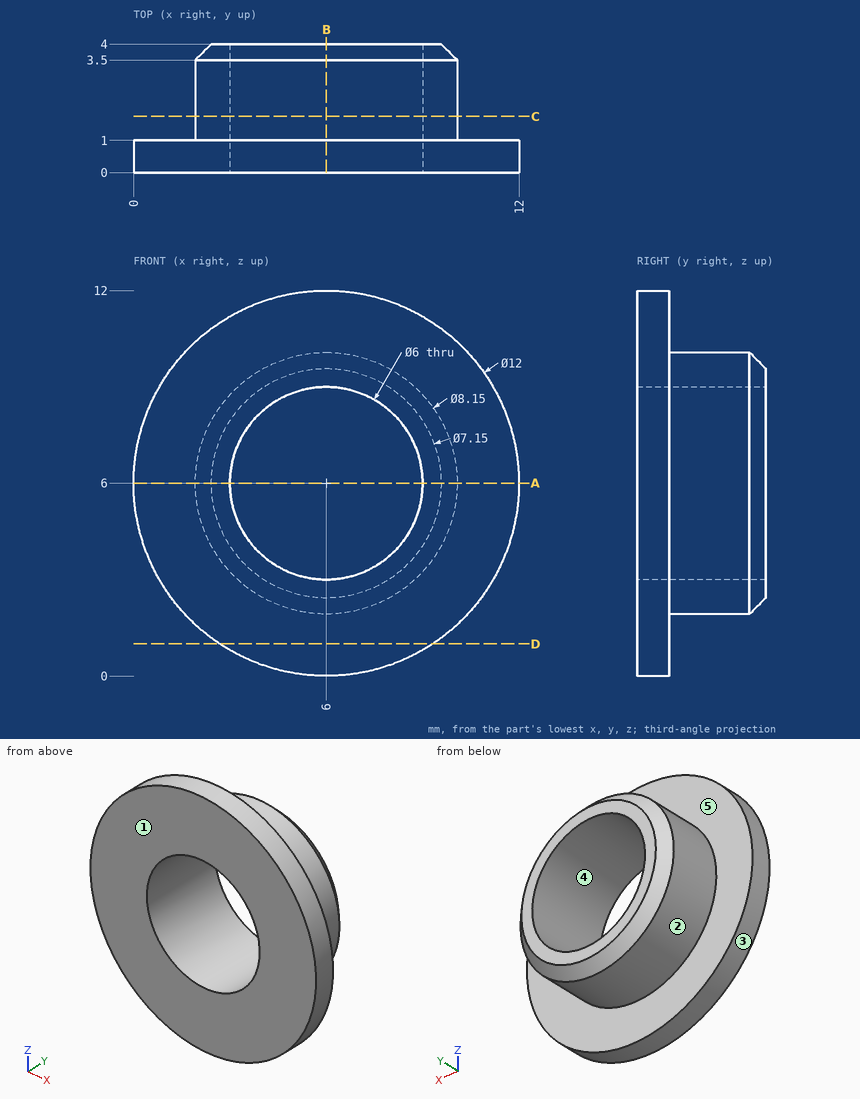
Geometry check sheet. Reference: drawing and pictorial views, mm from the part's lowest x, y, z. A direction names the side the tool comes from. Round coordinates to 2 decimals unless told otherwise and drop trailing zeros. Loops run counter-clockwise (first coordinate to the right, second up) from the corner with the lowest first, then second, coordinate; pieces in that order, holes last. Notation, with made-up numbers: (40.25, 45.5) -> (74.25, 45.5) arc R23 cw to (74.25, 58.5) -> close; hole circle Ø2 at (-34, 20.5). An arc over 180 degrees is marked (long way). Answer as a JSON object with one key per item and string values. Group by question number.
Item 1: Cross-section at C-C, the plane y = 1.75. Record the cut outline in (x, z) (3 decimals), plus the area to 3 significant figures.
Item 2: Cross-section at D-D, the plane z = 1. Record the cut outline in (x, y), plus the area to 3 significant figures.
Item 3: Set-up check for the marked faces 1 and 2: record each of +Z, -Z, +X, -X, +Y, -Y from which the full face is reachable in a straight line by a thin tool's end or side.
Item 4: Thickness scan on line 1 along X through (y, z) = (2.1, 6) (3 decimals); line 2 along Z through (x, y) = (4, 0.85); line 3 along X through (y, z) = (3.4, 3.5). Record the ranges inside material, lowest first.
Item 5: Release check for a two-part mould opening along X. For the marked faces 3, 4 and 5 record: pulls with the +X half, pulls with the -X half, needs draft (parallel to the pull), parting line crosses it, or undercut.
Item 6: Cross-section at B-B, the plane x = 6. Record the cut outline in (y, z) (3 decimals).
Item 7: Cross-section at A-A, the plane z = 6. Record the cut outline in (x, y) (3 decimals), plus the area to 3 significant figures.
Item 8: Depth check by flat-ended pin: pin 1 Ø2 at (x, y) = (5, 3) entering from +Z (3 decimals); pin 2 Ø2 at (y, z) = (1, 8) entering from +X; pin 3 Ø7 at (x, z) = (6, 6) entering from +Y. Enter the tip coordinate at first touch or a pass-through.
Determined:
{
 "1": {"outline": "circle Ø8.15 at (6, 6); hole circle Ø6 at (6, 6)", "area": "23.9 mm²"},
 "2": {"outline": "(2.68, 0) -> (9.32, 0) -> (9.32, 1) -> (2.68, 1) -> close", "area": "6.63 mm²"},
 "3": {"face 1": "+Z, -Z, +X, -X, -Y", "face 2": "+Y"},
 "4": {"line 1": "x = 1.925 to 3, 9 to 10.075", "line 2": "z = 0.34 to 3.76, 8.24 to 11.66", "line 3": "x = 2.78 to 4.34, 7.66 to 9.22"},
 "5": {"face 3": "parting line crosses it", "face 4": "undercut", "face 5": "needs draft"},
 "6": {"outline": "(0, 0) -> (1, 0) -> (1, 1.925) -> (3.5, 1.925) -> (4, 2.425) -> (4, 3) -> (0, 3) -> close; (0, 9) -> (4, 9) -> (4, 9.575) -> (3.5, 10.075) -> (1, 10.075) -> (1, 12) -> (0, 12) -> close"},
 "7": {"outline": "(0, 0) -> (3, 0) -> (3, 4) -> (2.425, 4) -> (1.925, 3.5) -> (1.925, 1) -> (0, 1) -> close; (9, 0) -> (12, 0) -> (12, 1) -> (10.075, 1) -> (10.075, 3.5) -> (9.575, 4) -> (9, 4) -> close", "area": "12.2 mm²"},
 "8": {"pin 1": "stops at z = 10.075", "pin 2": "stops at x = 11.92", "pin 3": "stops at y = 4"}
}
